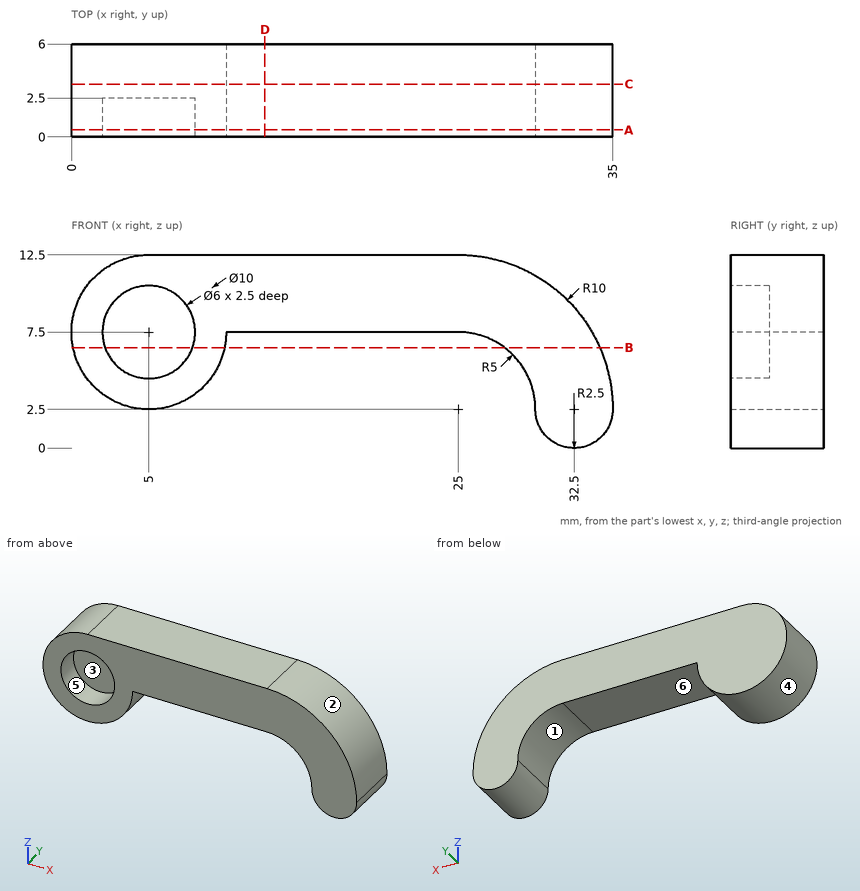
Study the drawing (mm; zero at the part's minimum x, y, z) and answer. A direction names the side the tool comes from. Give positions to 0.01 mm unless a question says otherwise; leave off trailing zeros. Loops run counter-clockwise (first coordinate to the right, second up) from the corner with the lowest first, then second, coordinate; pieces in that order, holes last. Notation, with made-up numbers: M 86.25,48.25 L 90.25,48.25 A13 ccw 90.25,71.25 Z; hole C -16.75,15 d9. An arc over 180 degrees is marked long. Answer as CSV lines item,"result".
Item 1: The part is cut by section D-D (x = 12.5). Give the vertices of the cut face in (y, z).
Values follow:
outline,"M 0,7.5 L 6,7.5 L 6,12.5 L 0,12.5 Z"
Item 2: The part is cut by section A-A (y = 0.45). Give the vertices of the cut face in (x, z), and give its area (3 significant figures).
Values follow:
outline,"M 5,12.5 A5 ccw long 10,7.5 L 25,7.5 A5 cw 30,2.5 A2.5 ccw 35,2.5 A10 ccw 25,12.5 Z; hole C 5,7.5 d6"
area,"199 mm^2"
Item 3: The mould has two halves that part along Z. Classify the marked faces 1, 2 and 3: released by +Z, released by -Z, zero draft, split by the parting line, or undercut.
Values follow:
face 1,"released by -Z"
face 2,"released by +Z"
face 3,"undercut"
Item 4: The part is cut by section B-B (z = 6.5). Give the vertices of the cut face in (x, y).
Values follow:
outline,"M 0.1,0 L 2.17,0 L 2.17,2.5 L 7.83,2.5 L 7.83,0 L 9.9,0 L 9.9,6 L 0.1,6 Z; M 28,0 L 34.17,0 L 34.17,6 L 28,6 Z"
Item 5: Which of the six approach directions +Z, -Z, +X, -X, +Y, -Y give full straight-line access (tool end or side, diameter ignored) to the marked faces 4, 5 and 6?
Values follow:
face 4,"+Y, -Y"
face 5,"-Y"
face 6,"-Z, +Y, -Y"
Item 6: The part is cut by section C-C (y = 3.4). Give the vertices of the cut face in (x, z).
Values follow:
outline,"M 5,12.5 A5 ccw long 10,7.5 L 25,7.5 A5 cw 30,2.5 A2.5 ccw 35,2.5 A10 ccw 25,12.5 Z"
Item 7: Straight lines are drawn through the part: line 1 along Y through (x, z) = (4, 7.25); line 2 along Z through (x, y) = (14, 4.25); line 3 along X through (y, z) = (3.9, 6.75). For each, find the intervals that lie inside material, in ascending order. Write a range as [from, to].
Values follow:
line 1,"y = [2.5, 6]"
line 2,"z = [7.5, 12.5]"
line 3,"x = [0.06, 9.94], [27.63, 34.05]"
Item 8: Given pin 1 Ø1.5 at (y, z) = (2, 9.5) entering from -X; pin 2 Ø1 at (y, z) = (2.5, 11) entering from +X; pin 3 Ø2 at (x, y) = (25.5, 1) entering from -Z, each flat-ended and moving along its own axis, determine where each tip first touches the part or whether it passes through.
Values follow:
pin 1,"stops at x = 0.16"
pin 2,"stops at x = 31"
pin 3,"stops at z = 7.27"
